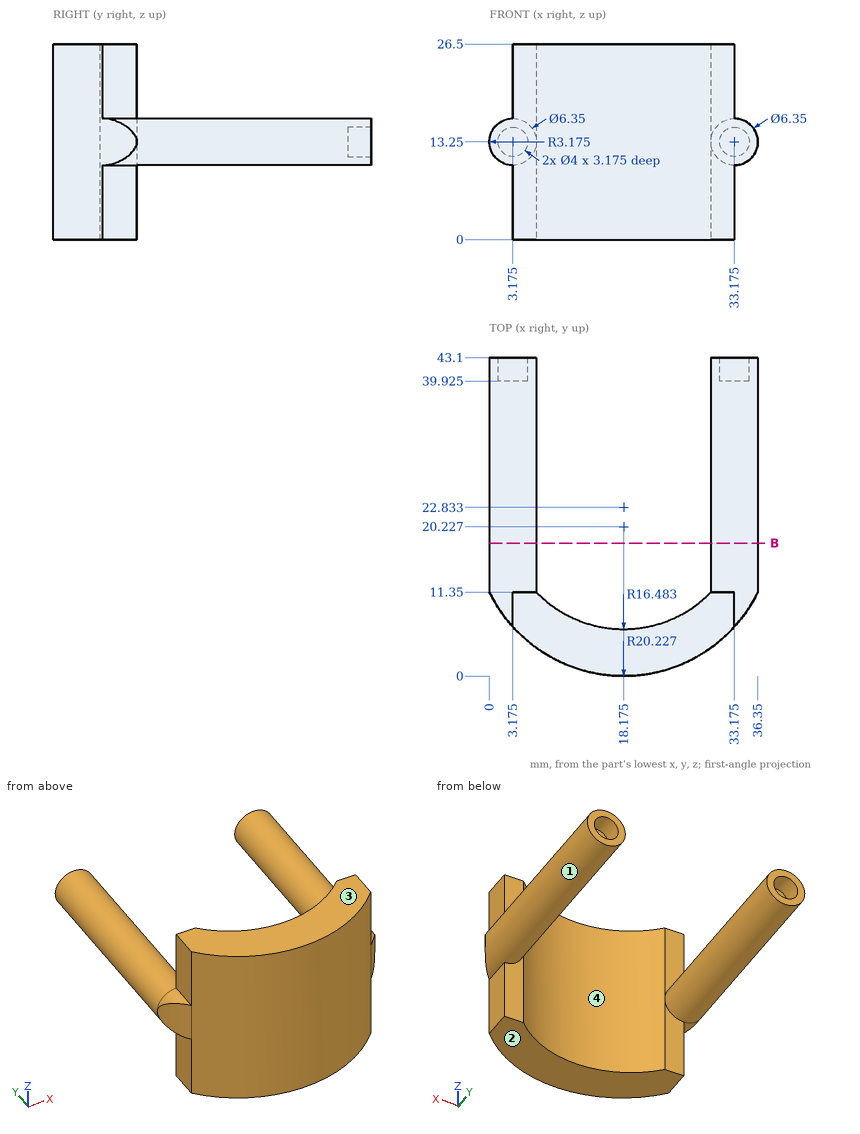
Study the drawing (mm; zero at the part's minimum x, y, z) and answer. A direction names the side the tool comes from. Round coordinates to 2 decimals unless told otherwise and drop trailing zeros. Order: outer loops, then holes, each group sorted by start corner. A loop starts at its lowest first (then second) coordinate and runs counter-clockwise, first axis right, second up. Notation, with made-up numbers: (-20.75, 84) -> (-7.75, 84) arc R12 ccw to (-7.75, 92) -> close; hole circle Ø11 at (76, -4). An arc over 180 degrees is marked (long way). Answer as CSV lines item,"result". Start each with the question number.
(1) Find the intervals of material crossed by probe 1 along X at (y, z) = (41.95, 13.25) (3 decimals); probe 2 along X at (y, z) = (10, 7) (1 decimal); probe 3 along X at (y, z) = (26, 15.75), in increasing order. Write a range as from..to.
(2) Flat-ended cylindrical pins translate along their axes: pin 1 Ø2 at (x, z) = (4, 12.5) entering from +Y; pin 2 Ø5 at (x, z) = (25.5, 6.5) entering from +Y; pin 3 Ø2.5 at (y, z) = (8.5, 2.5) entering from +X (3 decimals); pin 4 Ø2.5 at (x, z) = (3.175, 13.25) entering from -Y. Find the tip coordinate at first contact, or state that the pin passes through.
(3) A tool of negligible diameter and unlimited length cuts with its end or side. For the marked faces 1 and 2, from which of +Z, -Z, +X, -X, +Y, -Y can it reach the whole face along a straight path? Write none if from no direction.
(4) The part is cut by section B-B (y = 18). Determine the outline of the cut face in (x, z) (3 decimals).
(5) For a pull along X with two mould halves and no side action, classify the marked faces 3 and 4 as +X half, -X half, draft (parallel to the pull), parting line (faces both ways), or undercut.
Evaluation:
1,probe 1,"0..1.175, 5.175..6.35, 30..31.175, 35.175..36.35"
1,probe 2,"3.2..7.8, 28.5..33.2"
1,probe 3,"1.22..5.13, 31.22..35.13"
2,pin 1,"y = 43.1"
2,pin 2,"y = 9.6"
2,pin 3,"x = 33.175"
2,pin 4,"y = 5.39"
3,face 1,"+Y"
3,face 2,"-Z, +X, -X, +Y, -Y"
4,outline,"circle Ø6.35 at (3.175, 13.25); circle Ø6.35 at (33.175, 13.25)"
5,face 3,"draft"
5,face 4,"undercut"
